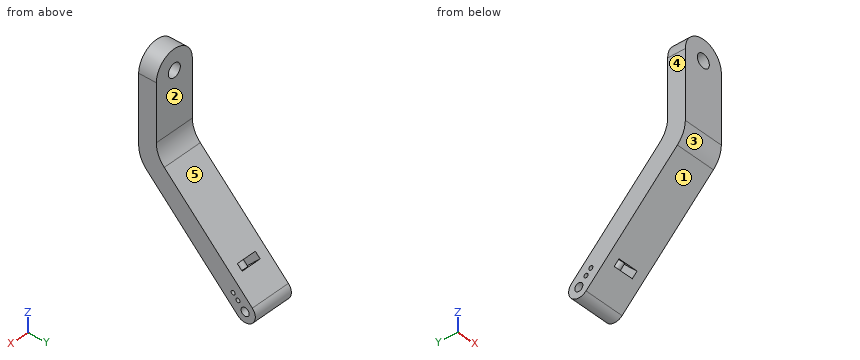
Autodesk Inventor part; units mm, degrees
ref_plane "YZ Plane" through (0, 0, 0) normal (1, 0, 0) x (0, 1, 0)
ref_plane "XZ Plane" through (0, 0, 0) normal (0, 1, 0) x (-1, 0, 0)
ref_plane "XY Plane" through (0, 0, 0) normal (0, 0, 1) x (1, 0, 0)
sketch "草圖1" plane through (0, 0, 0) normal (0, 1, 0) x (-1, 0, 0)
  line L0 (0, 150) -> (-300, 150)
  line L1 (-300, 0) -> (-300, 150)
  arc A0 (-300, 0) -> (0, 0) centre (-150, 0) ccw
  line L2 (0, 150) -> (0, 0)
  line L3 (0, 271.7864) -> (0, 150)
  line L4 (-300, 271.7864) -> (0, 271.7864)
  line L5 (-300, 150) -> (-300, 271.7864)
  circle A1 centre (-150, 0) radius 50
  line L6 (-30.3819, -276.523) -> (-200, -276.523)
  line L7 (0, -703.0461) -> (-300, -703.0461)
  line L8 (-300, -553.0461) -> (-300, -703.0461)
  arc A2 (0, -553.0461) -> (-300, -553.0461) centre (-150, -553.0461) ccw
  line L9 (0, -703.0461) -> (0, -553.0461)
  circle A3 centre (-150, -553.0461) radius 50
extrude "擠出1" add sketch "草圖1" along normal blind 130 contours L7 L8 A2 L9
ref_plane "工作平面1" through (150, 0, -553.0461) normal (1, 0, 0) x (0, 0, -1)
sketch "草圖2" plane through (150, 0, -553.0461) normal (1, 0, 0) x (0, 0, -1)
  line L0 (-150, 0) -> (-150, 130)
  line L1 (-150, 130) -> (-50, 130)
  line L2 (-50, 130) -> (-50, 0)
  line L3 (-50, 0) -> (-150, 0)
  line L4 (150, 130) -> (150, 0)
  line L5 (150, 0) -> (50, 0)
  line L6 (50, 0) -> (50, 130)
  line L7 (50, 130) -> (150, 130)
  line L8 (150, 0) -> (150, 130)
  line L9 (150, 130) -> (500, 130)
  line L10 (500, 130) -> (500, 0)
  line L11 (500, 0) -> (150, 0)
  line L12 (150, 0) -> (150, 130)
  line L13 (150, 130) -> (0, 130)
  line L14 (500, 130) -> (606.066, 23.934)
  line L15 (606.066, 23.934) -> (1313.1728, 731.0408)
  line L16 (1313.1728, 731.0408) -> (1207.1068, 837.1068)
  line L17 (1207.1068, 837.1068) -> (500, 130)
  line L18 (606.066, 23.934) -> (582.132, 0)
  line L19 (500, 0) -> (582.132, 0)
  circle A0 centre (1260.1398, 784.0738) radius 75
  circle A1 centre (1207.1068, 731.0408) radius 15
  line L20 (1260.1398, 784.0738) -> (1207.1068, 731.0408)
  circle A2 centre (1260.1398, 784.0738) radius 30
  circle A3 centre (1171.7514, 695.6854) radius 15
  line L21 (1207.1068, 731.0408) -> (1171.7514, 695.6854)
  point P0 (-553.0461, 0)
  point P1 (1313.1728, 731.0408)
  dimension "d2" = 500
  dimension "d3" = 1000
  dimension "d4" = 150
  dimension "d5" = 45
  dimension "d6" = 30
  dimension "d7" = 60
  dimension "d8" = 30
  dimension "d9" = 50
extrude "擠出2" add sketch "草圖2" along normal mid plane 300 contours L9 L10 L11 L4 | L14 L18 L19 L10 | L17 A0 A1 L15 L14 | A0 L16 A2 | L16 A2 L20 A1 A0 | A0 A1 L20 A2 L16
sketch "草圖3" plane through (0, 130, -1053.0461) normal (0, 0.7071, 0.7071) x (1, 0, 0)
  line L0 (0, -183.8478) -> (0, 0)
  line L1 (0, 0) -> (0, 1000)
  line L2 (0, 1000) -> (300, 1000)
  line L3 (300, 1000) -> (300, 0)
  line L4 (0, 0) -> (300, 0)
  line L5 (300, -183.8478) -> (0, -183.8478)
  line L6 (300, 0) -> (300, -183.8478)
  line L7 (75, 800) -> (225, 800)
  line L8 (225, 800) -> (225, 750)
  line L9 (225, 750) -> (75, 750)
  line L10 (75, 750) -> (75, 800)
  point P0 (0, -836.5399)
  point P1 (150, 800)
  point P2 (150, 1000)
  dimension "d12" = 200
  dimension "d13" = 50
  dimension "d14" = 150
extrude "擠出3" cut sketch "草圖3" against normal blind 300 contours L7 L8 L9 L10
fillet "圓角1" radius 200 2 edges at (150, 130, -1053.0461) (150, 0, -1135.1781)
sketch "草圖4" plane through (225, 660.3301, -1583.3761) normal (0, 0.7071, -0.7071) x (-1, 0, 0)
  line L0 (225, -150) -> (150, -150)
  line L1 (150, -150) -> (0, -150)
  line L2 (0, -150) -> (-75, -150)
  line L3 (-75, -150) -> (-75, 0)
  line L4 (-75, 0) -> (0, 0)
  line L5 (0, 0) -> (0, -150)
  line L6 (225, 0) -> (225, -150)
  line L7 (150, 0) -> (225, 0)
  line L8 (0, 0) -> (150, 0)
  line L9 (150, -150) -> (150, 0)
  circle A0 centre (75, -75) radius 25
  point P0 (225, 652.6921)
  point P1 (75, 0)
  point P2 (0, -75)
  dimension "d18" = 50
extrude "擠出4" add sketch "草圖4" along normal up to next contours A0
equation "\"d8\" = d6"
properties part number "主吊臂"
Check sheet for the modelled part. Datum: model origin and axes. Units: mm. Face numbers are marked on the shaded views. A direction names the side the tool comes from. Coordinates: 2 decimals unless noted, no trailing zeros. Write each loop counter-clockwise with the first axis right and the second up, starting at its lowest first coordinate (ties: lowest second). Pieces come first, ordered by that corner, then holes. Notation, with made-up numbers: (84, 5.5) - (97, 5.5) arc R20 ccw to (97, 11.5) - close; hole circle Ø5 at (60, 6). An arc over 180 degrees is marked (long way). One line per question, with ' | ' between items.
Item 1: Access from +Z, -Z, +X, -X, +Y, -Y to the whole of each face (thin tool, end or side, straight path). Record for the marked faces 1 and 2.
Determined:
face 1: -Z, +X, -X, -Y | face 2: +Z, +X, -X, +Y
Item 2: Gauge pin test, flat ends, axial feed: P1, Ø5, axis at x = 215, y = 271.5, coming from the +Z side; P2, Ø6, axis at x = 51, z = -733.5, coming from the +Y side; P3, Ø6, axis at x = 244, y = 158, coming from the -Z side. Record the tip position at first contact, or that the pin passes through.
Determined:
P1: stops at z = -1192.05 | P2: stops at y = 130 | P3: stops at z = -1296.18
Item 3: Sectioned sample at A-A on x = 150. Record the boundary of the cut face in (y, z).
Determined:
outline: (0, -1052.34) arc R200 ccw to (58.58, -1193.76) - (554.26, -1689.44) - (589.62, -1654.09) - (624.97, -1689.44) - (589.62, -1724.8) - (731.04, -1866.22) arc R75 ccw to (837.11, -1760.15) - (695.69, -1618.73) - (660.33, -1654.09) - (624.97, -1618.73) - (660.33, -1583.38) - (188.58, -1111.62) arc R200 cw to (130, -970.2) - (130, -603.05) - (0, -603.05) - close; (0, -503.05) - (130, -503.05) - (130, -403.05) - (0, -403.05) - close; hole circle Ø30 at (695.69, -1724.8); hole circle Ø30 at (731.04, -1760.15); hole circle Ø60 at (784.07, -1813.19)
Item 4: Thickness scan on line 1 (Z direction, x = 207.5, y = 610.5); line 2 (Z direction, x = 123.5, y = 729); line 3 (X direction, y = 53, z = -589). Record the ranges inside material, lowest first. Write a range as [from, to].
Determined:
line 1: z = [-1745.68, -1703.92], [-1633.21, -1533.55] | line 2: z = [-1864.18, -1775.01], [-1745.29, -1652.05] | line 3: x = [0, 115.25], [184.75, 300]
Item 5: Mould release check, pull along Y, two halves, no side actions. Record for the marked faces 3, 4 and 5: pulls with the +Y half, pulls with the -Y half, needs draft (parallel to the pull), parting line crosses it, or undercut.
Determined:
face 3: pulls with the -Y half | face 4: needs draft | face 5: pulls with the +Y half
Item 6: Sectioned sample at C-C on z = -1093.5. Record the boundary of the cut face in (x, y), plus the area to 3 significant figures.
Determined:
outline: (0, 4.28) - (300, 4.28) - (300, 172.53) - (0, 172.53) - close | area: 50,500 mm2
Item 7: Sectioned sample at B-B on x = 51. Record the boundary of the cut face in (y, z), plus the area to 3 significant figures.
Determined:
outline: (0, -1052.34) arc R200 ccw to (58.58, -1193.76) - (731.04, -1866.22) arc R75 ccw to (837.11, -1760.15) - (188.58, -1111.62) arc R200 cw to (130, -970.2) - (130, -440.36) - (0, -440.36) - close; hole circle Ø30 at (695.69, -1724.8); hole circle Ø30 at (731.04, -1760.15); hole circle Ø60 at (784.07, -1813.19) | area: 242,000 mm2
Item 8: Sectioned sample at D-D on x = 248. Record the boundary of the cut face in (y, z), plus the area to 3 significant figures.
Determined:
outline: (0, -1052.34) arc R200 ccw to (58.58, -1193.76) - (731.04, -1866.22) arc R75 ccw to (837.11, -1760.15) - (188.58, -1111.62) arc R200 cw to (130, -970.2) - (130, -439.49) - (0, -439.49) - close; hole circle Ø30 at (695.69, -1724.8); hole circle Ø30 at (731.04, -1760.15); hole circle Ø60 at (784.07, -1813.19) | area: 242,000 mm2
